Design review of the part built by this model. Coordinates are the model's own, in mm. Face numbers are marked on the shaded views. A direction names the side the tool comes from. Give positions to 0.01 mm unless a question says otherwise; leave off trailing zeros. Write each loop counter-clockwise with the first axis right and the second up, starting at its lowest first coordinate (ties: lowest second). Pieces come first, ordered by that corner, then holes. Notation, with made-up numbers: M -20.75,-22.75 L 12.25,-22.75 A28 cw 12.25,16.25 Z; hole C 9.5,-35 d9. An arc over 180 degrees is marked long. Answer in a Markdown table with one row per item.
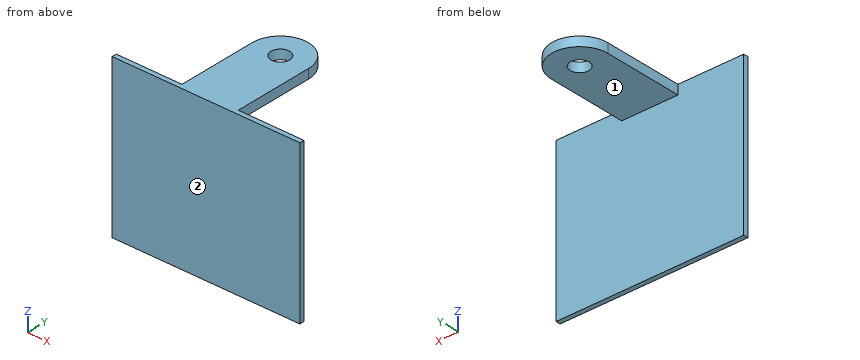
Autodesk Inventor part; units mm, degrees
ref_plane "YZ Plane" through (0, 0, 0) normal (1, 0, 0) x (0, 1, 0)
ref_plane "XZ Plane" through (0, 0, 0) normal (0, 1, 0) x (-1, 0, 0)
ref_plane "XY Plane" through (0, 0, 0) normal (0, 0, 1) x (1, 0, 0)
sketch "草圖1" plane through (0, 0, 0) normal (0, 0, 1) x (1, 0, 0)
  line L0 (0, 0) -> (0, -85) construction
  line L1 (-30, 0) -> (-30, -85)
  line L2 (30, -85) -> (30, 0)
  arc A0 (30, 0) -> (-30, 0) centre (0, 0) ccw
  arc A1 (-30, -85) -> (30, -85) centre (0, -85) ccw construction
  line L3 (-30, -85) -> (30, -85)
  point P0 (0, -42.5)
  dimension "d0" = 30
  dimension "d1" = 85
extrude "擠出1" add sketch "草圖1" along normal blind 10
sketch "草圖2" plane through (0, 0, 0) normal (0, 0, -1) x (-1, 0, 0)
  arc A0 (30, 0) -> (-30, 0) centre (0, 0) ccw
  circle A1 centre (0, 0) radius 10
  dimension "d4" = 20
extrude "擠出2" cut sketch "草圖2" against normal blind 10
sketch "草圖3" plane through (-30, -85, 0) normal (0, -1, 0) x (1, 0, 0)
  line L0 (0, 10) -> (60, 10)
  line L1 (-70, 10) -> (130, 10)
  line L2 (130, 10) -> (130, -160)
  line L3 (130, -160) -> (-70, -160)
  line L4 (-70, -160) -> (-70, 10)
  point P0 (30, 0)
  dimension "d7" = 100
  dimension "d8" = 200
  dimension "d9" = 170
extrude "擠出3" add sketch "草圖3" along normal blind 5
1) Add section A-A (x = 0). Write out the cut boundary in (y, z).
Geometry says:
| item | result |
|---|---|
| outline | M -90,-160 L -85,-160 L -85,0 L -10,0 L -10,10 L -90,10 Z; M 10,0 L 30,0 L 30,10 L 10,10 Z |
2) Add section C-C (y = -32.5). Write out the cut boundary in (x, z), and give its area (3 significant figures).
Geometry says:
| item | result |
|---|---|
| outline | M -30,0 L 30,0 L 30,10 L -30,10 Z |
| area | 600 mm^2 |
3) For the marked faces 1 and 2, list the 3-axis set-ups (+Z, -Z, +X, -X, +Y, -Y) from which the entire face can be reached by the end or side of a thin tool; tool diameter is ignored.
Geometry says:
| item | result |
|---|---|
| face 1 | -Z, +X, -X, +Y |
| face 2 | +Z, -Z, +X, -X, -Y |
4) Add section B-B (z = -46.5). Write out the cut boundary in (x, y), and give its area (3 significant figures).
Geometry says:
| item | result |
|---|---|
| outline | M -100,-90 L 100,-90 L 100,-85 L -100,-85 Z |
| area | 1,000 mm^2 |
5) Insertion check: P1, Ø11, axis at y = -38.5, z = 5.5, coming from the -X side; P2, Ø1.5, axis at x = 30.5, z = -53, coming from the +Y side; P3, Ø3, axis at y = -37, z = 7, coming from the +X side. Each pin has a flat end and moves straight along its axis. Give the tip position at first contact, or say it passes through.
Geometry says:
| item | result |
|---|---|
| P1 | x = -30 |
| P2 | y = -85 |
| P3 | x = 30 |
6) Add section D-D (x = 25.5). Write out the cut boundary in (y, z), and give its area (3 significant figures).
Geometry says:
| item | result |
|---|---|
| outline | M -90,-160 L -85,-160 L -85,0 L 15.8,0 L 15.8,10 L -90,10 Z |
| area | 1,860 mm^2 |
7) To check wall thickness, follow probe 1 along Y at (x, z) = (0, 4.25); probe 2 along Y at (x, z) = (-5, -33.5); probe 3 along Z at (x, y) = (-20, -54). State the ranges of each line that lie inside material, in increasing order. Write a range as [from, to].
Geometry says:
| item | result |
|---|---|
| probe 1 | [-90, -10], [10, 30] |
| probe 2 | [-90, -85] |
| probe 3 | [0, 10] |
